Work out the finished part from the listing and answer in its coordinate system (mm). A direction names the side the tool comes from. Give positions to 0.01 mm unless a question says otherwise; leave off trailing zeros. Order: outer loops, then holes, each group sorted by start corner. A loop starts at its lowest first (then second) coordinate and runs counter-clockwise, first axis right, second up. Notation, with made-up numbers: (37, -27) -> (42, -27) arc R11 ccw to (42, -16) -> close; hole circle Ø1 at (67, 36.5). An arc over 180 degrees is marked (long way). Answer as CSV lines item,"result". Start each with the question number.
1. A cutting plane is placed at B-B (z = 11.5). Give the vertices of the cut face in (x, y) (3 decimals).
2. For a pull along Y with two mould halves and no side action, classify faces 1 (the flat face through (46, 25.4, 13)), 2 (the cylindrical face through (-15.12, -11.59, 37.92)), 3 (the flat face through (-48, -25.4, 13)) as released by +Y, released by -Y, zero draft, split by the parting line, or undercut.
3. Flat-ended cylindrical pins translate along their axes: pin 1 (12 mm diameter, centred on x = -20.5, y = 25.5, fed in from +Z); pin 2 (5 mm diameter, centred on y = -8.5, z = 12.5, fed in from -X); pin 3 (12 mm diameter, centred on x = 77, y = 17.5, fed in from +Z); pin 4 (12 mm diameter, centred on y = 21.5, z = 32.5, fed in from +X). Find the tip coordinate at first contact, or state that the pin passes through.
4. For faces 4 (the flat face through (46, -25.4, 13)), 5 (the flat face through (59, -9.525, 13)), 6 (the flat face through (4, -12.4, 25.4)), determine the directions among +Z, -Z, +X, -X, +Y, -Y from which every point of the face is accessible in a straight line to the end or side of a thin tool.
5. A cutting plane is placed at D-D (y = -23). Give the vertices of the cut face in (x, z), then the cut area to 3 significant figures.
6. A cutting plane is placed at A-A (x = 0). Give the vertices of the cut face in (y, z).
7. A cutting plane is placed at C-C (y = -3). Give the vertices of the cut face in (x, z).
8. Find the intervals of material crossed by L1, parallel to Y at x = 0, z = 9.75; L2, parallel to X at y = 7, z = 17; L3, parallel to Y at x = 0, z = 44, in increasing order.
from build123d import *

# Parameters (mm, degrees)
F0_R     = 19.05
F1_DEPTH = 50.8
F0_R_2   = 9.525
F2_DEPTH = 25.4
F3_DEPTH = 25.4
F0_R_3   = 12.7
F4_DEPTH = 25.4


with BuildPart() as f1:
    # F0 (on Top) → F1 (new body)
    with BuildSketch(Plane.XY):
        with BuildLine():
            ThreePointArc((19.05, -25.4), (28.398063, -14.199032), (31.75, 0))
            ThreePointArc((31.75, 0), (28.398063, 14.199032), (19.05, 25.4))
            ThreePointArc((19.05, 25.4), (0, 31.75), (-19.05, 25.4))
            ThreePointArc((-19.05, 25.4), (-31.75, 0), (-19.05, -25.4))
            ThreePointArc((-19.05, -25.4), (0, -31.75), (19.05, -25.4))
        make_face()
        Circle(F0_R, mode=Mode.SUBTRACT)
    extrude(amount=F1_DEPTH)

    # F0 (on Top) → F2 (join)
    with BuildSketch(Plane.XY):
        with BuildLine():
            ThreePointArc((-19.05, -25.4), (-31.75, 0), (-19.05, 25.4))
            Line((-19.05, 25.4), (-76.161206, 25.4))
            ThreePointArc((-76.161206, 25.4), (-101.561206, 0), (-76.161206, -25.4))
            Line((-76.161206, -25.4), (-19.05, -25.4))
        make_face()
        with Locations((-76.161206, 0)):
            Circle(F0_R_2, mode=Mode.SUBTRACT)
    extrude(amount=F2_DEPTH)

    # F0 (on Top) → F3 (join)
    with BuildSketch(Plane.XY):
        with BuildLine():
            ThreePointArc((19.05, 25.4), (28.398063, 14.199032), (31.75, 0))
            ThreePointArc((31.75, 0), (28.398063, -14.199032), (19.05, -25.4))
            Line((19.05, -25.4), (73.097611, -25.4))
            ThreePointArc((73.097611, -25.4), (98.497611, 0), (73.097611, 25.4))
            Line((73.097611, 25.4), (19.05, 25.4))
        make_face()
        with BuildLine():
            ThreePointArc((73.097611, 9.525), (82.622611, 0), (73.097611, -9.525))
            Line((73.097611, -9.525), (45.157611, -9.525))
            ThreePointArc((45.157611, -9.525), (35.632611, 0), (45.157611, 9.525))
            Line((45.157611, 9.525), (73.097611, 9.525))
        make_face(mode=Mode.SUBTRACT)
    extrude(amount=F3_DEPTH)

    # F0 (on Top) → F4 (join)
    with BuildSketch(Plane.XY):
        Circle(F0_R)
        Circle(F0_R_3, mode=Mode.SUBTRACT)
    extrude(amount=F4_DEPTH)


solid = f1.part
Answer sheet:
1,outline,"(-76.161, -25.4) -> (-19.05, -25.4) arc R31.75 ccw to (19.05, -25.4) -> (73.098, -25.4) arc R25.4 ccw to (73.098, 25.4) -> (19.05, 25.4) arc R31.75 ccw to (-19.05, 25.4) -> (-76.161, 25.4) arc R25.4 ccw to start; hole circle Ø19.05 at (-76.161, 0); hole circle Ø25.4 at (0, 0); hole (45.158, -9.525) -> (73.098, -9.525) arc R9.525 ccw to (73.098, 9.525) -> (45.158, 9.525) arc R9.525 ccw to start"
2,face 1,"released by +Y"
2,face 2,"undercut"
2,face 3,"released by -Y"
3,pin 1,"stops at z = 50.8"
3,pin 2,"stops at x = -100.84"
3,pin 3,"stops at z = 25.4"
3,pin 4,"stops at x = 27.71"
4,face 4,"+Z, -Z, +X, -Y"
4,face 5,"+Z, -Z"
4,face 6,"+Z"
5,outline,"(-86.94, 0) -> (83.88, 0) -> (83.88, 25.4) -> (21.89, 25.4) -> (21.89, 50.8) -> (-21.89, 50.8) -> (-21.89, 25.4) -> (-86.94, 25.4) -> close"
5,area,"5,450 mm^2"
6,outline,"(-31.75, 0) -> (-12.7, 0) -> (-12.7, 25.4) -> (-19.05, 25.4) -> (-19.05, 50.8) -> (-31.75, 50.8) -> close; (12.7, 0) -> (31.75, 0) -> (31.75, 50.8) -> (19.05, 50.8) -> (19.05, 25.4) -> (12.7, 25.4) -> close"
7,outline,"(-101.38, 0) -> (-85.2, 0) -> (-85.2, 25.4) -> (-101.38, 25.4) -> close; (-67.12, 0) -> (-12.34, 0) -> (-12.34, 25.4) -> (-18.81, 25.4) -> (-18.81, 50.8) -> (-31.61, 50.8) -> (-31.61, 25.4) -> (-67.12, 25.4) -> close; (12.34, 0) -> (36.12, 0) -> (36.12, 25.4) -> (31.61, 25.4) -> (31.61, 50.8) -> (18.81, 50.8) -> (18.81, 25.4) -> (12.34, 25.4) -> close; (82.14, 0) -> (98.32, 0) -> (98.32, 25.4) -> (82.14, 25.4) -> close"
8,L1,"y = -31.75 to -12.7, 12.7 to 31.75"
8,L2,"x = -100.58 to -82.62, -69.7 to -10.6, 10.6 to 38.7, 79.56 to 97.51"
8,L3,"y = -31.75 to -19.05, 19.05 to 31.75"
